```python
from build123d import *

# Parameters (mm, degrees)
BOSS_EXTRU_1_DEPTH      = 5
ESQUISSE2_W             = 5
ESQUISSE2_H             = 5
ENL_V_MAT_EXTRU_1_DEPTH = 5


with BuildPart() as part:
    # Esquisse1 → Boss.-Extru.1 (new body)
    with BuildSketch(Plane.XY):
        Polygon((0, 0), (0, -19.685), (20, -19.685), (20, 4.433365096), (-55.2, 17.693154046), (-55.2, -19.685), (-40.2, -19.685), (-40.2, 0), align=None)
    extrude(amount=BOSS_EXTRU_1_DEPTH)

    # Esquisse2 → Enlèv. mat.-Extru.1 (cut)
    with BuildSketch(Plane(origin=(0, 0, 0), x_dir=(-1, 0, 0), z_dir=(0, 0, -1))):
        with BuildLine():
            Line((-10.537175757, 6.101916324), (-11.23314954, 10.048979788))
            Line((-11.23314954, 10.048979788), (-30.732234233, 6.610765057))
            Line((-30.732234233, 6.610765057), (-25.732815565, -21.742347141))
            Line((-25.732815565, -21.742347141), (-14.065020128, -19.685))
            ThreePointArc((-14.065020128, -19.685), (-15.760051103, -6.318330994), (-10.537175757, 6.101916324))
        make_face()
        with Locations((-10.5, -15.0925)):
            Rectangle(ESQUISSE2_W, ESQUISSE2_H)
    extrude(amount=-ENL_V_MAT_EXTRU_1_DEPTH, mode=Mode.SUBTRACT)


solid = part.part
```
The listing builds one solid part. Answer for the finished solid, in the listing's coordinates (mm). A direction names the side the tool comes from. Give positions to 0.01 mm unless a question says otherwise; leave off trailing zeros. Loops run counter-clockwise (first coordinate to the right, second up) from the corner with the lowest first, then second, coordinate; pieces in that order, holes last. Notation, with made-up numbers: (-29.75, -28.75) - (-15.75, -28.75) arc R36 ccw to (-15.75, 6.25) - close; hole circle Ø4 at (79.5, 70). An arc over 180 degrees is marked (long way). Return JSON: item names as keys, results as strings. Group by question number.
1. Find section B-B (y = -7). Write down the section's boundary in (x, z).
2. Given pin 1 Ø2.5 at (x, z) = (-12.5, 1.5) entering from -Y, flat-ended and moving along its own axis, determine where the tip first touches the part or whether it passes through.
3. Which of the six approach directions +Z, -Z, +X, -X, +Y, -Y give full straight-line access (tool end or side, diameter ignored) to faces 1 (the flat face through (-40.2, -10, 2)), 2 (the flat face through (7, -19.685, 2)), 3 (the flat face through (8, -15, 2))?
4. Determine the mould class of faces 4 (the flat face through (13, -15, 2)), 5 (the flat face through (-21.871, 11.816, 2.465)), 6 (the flat face through (-48, -19.685, 2)) for opening direction X: pulls with the +X half, pulls with the -X half, needs draft (parallel to the pull), parting line crosses it, or undercut.
5. Find section C-C (y = -11). Write down the section's boundary in (x, z).
6. Find section A-A (z = 4.05). Write down the section's boundary in (x, y) (1 decimal), then the cut area to 3 significant figures.
7. Straight lines are drawn through the part: line 1 (X direction, y = -15, z = 2.2); line 2 (X direction, y = -4, z = 3.2); line 3 (X direction, y = -16, z = 0.9). For each, find the intervals that lie inside material, in ascending order. Write a range as [from, to].
8. Find section D-D (x = -31). Write down the section's boundary in (y, z), then the cut area to 3 significant figures.
Verdict:
{
 "1": {"outline": "(-55.2, 0) - (-40.2, 0) - (-40.2, 5) - (-55.2, 5) - close; (0, 0) - (15.84, 0) - (15.84, 5) - (0, 5) - close"},
 "2": {"pin 1": "stops at y = 0"},
 "3": {"face 1": "+Z, -Z, -Y", "face 2": "+Z, -Z, +X, -X, -Y", "face 3": "+Z, -Z"},
 "4": {"face 4": "undercut", "face 5": "pulls with the +X half", "face 6": "needs draft"},
 "5": {"outline": "(-55.2, 0) - (-40.2, 0) - (-40.2, 5) - (-55.2, 5) - close; (0, 0) - (15.97, 0) - (15.97, 5) - (0, 5) - close"},
 "6": {"outline": "(-55.2, -19.7) - (-40.2, -19.7) - (-40.2, 0) - (0, 0) - (0, -19.7) - (14.1, -19.7) arc R26 ccw to (10.5, 6.1) - (-55.2, 17.7) - close; hole (8, -17.6) - (13, -17.6) - (13, -12.6) - (8, -12.6) - close", "area": "1,370 mm^2"},
 "7": {"line 1": "x = [-55.2, -40.2], [0, 8], [13, 15.48]", "line 2": "x = [-55.2, -40.2], [0, 15.34]", "line 3": "x = [-55.2, -40.2], [0, 8], [13, 15.26]"},
 "8": {"outline": "(0, 0) - (13.43, 0) - (13.43, 5) - (0, 5) - close", "area": "67.1 mm^2"}
}
